Check sheet for the drawn part. Datum: minimum x, y, z corner. Units: mm. A direction names the side the tool comes from. Give positions to 0.01 mm unless a question says otherwise; leave off trailing zeros. Write each loop counter-clockwise with the first axis right and the second up, starting at its lowest first coordinate (ties: lowest second). Pieces come first, ordered by that corner, then holes. Notation, with made-up numbers: (66.5, 31.25) - (117.5, 31.25) arc R30 ccw to (117.5, 61.25) - close; hole circle Ø10 at (-26, 16). An arc over 180 degrees is marked (long way). Use a Markdown table: item, result.
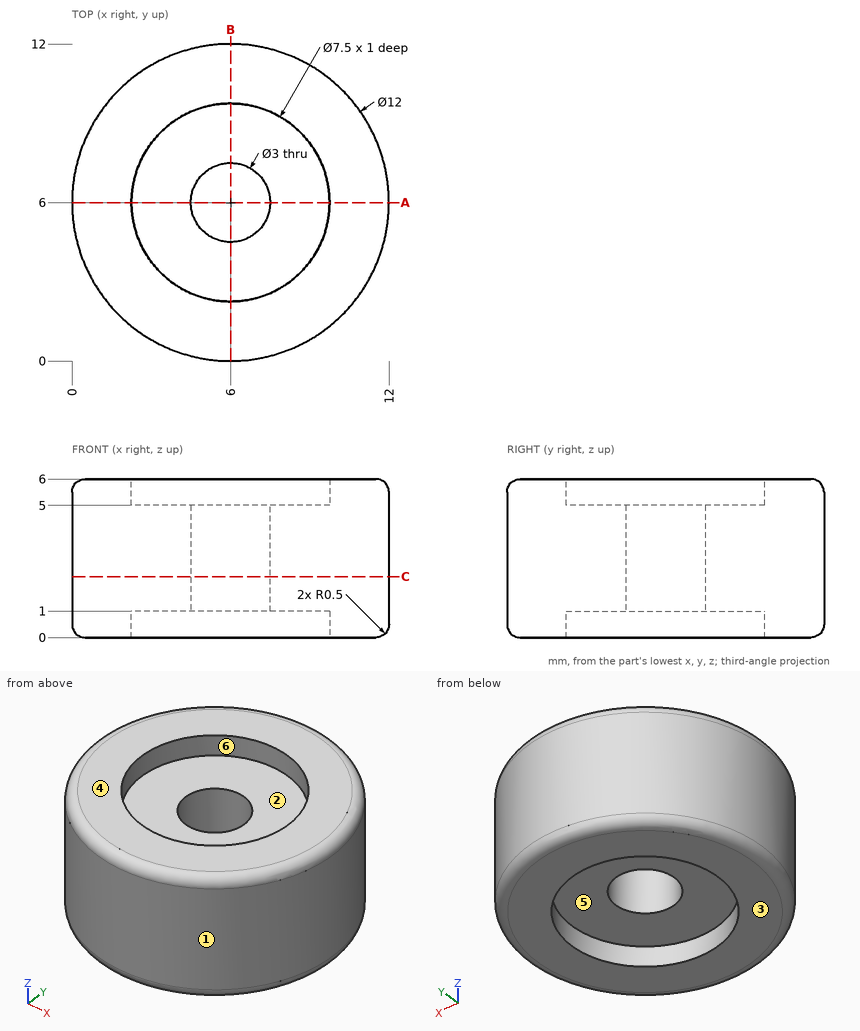
1) Material ranges on L1, parallel to Y at x = 6, z = 0.7; L2, parallel to Y at x = 6, z = 2.5; L3, parallel to Z at x = 9, y = 5.5, recorded low to high. Write a range as from..to.
Working result:
| item | result |
|---|---|
| L1 | y = 0..2.25, 9.75..12 |
| L2 | y = 0..4.5, 7.5..12 |
| L3 | z = 1..5 |
2) Mould release check, pull along X, two halves, no side actions. Record for the marked faces 1, 2 and 3: pulls with the +X half, pulls with the -X half, needs draft (parallel to the pull), parting line crosses it, or undercut.
Working result:
| item | result |
|---|---|
| face 1 | parting line crosses it |
| face 2 | undercut |
| face 3 | needs draft |
3) Section check A-A on y = 6. Record the boundary of the cut face in (x, z).
Working result:
| item | result |
|---|---|
| outline | (0, 0.5) arc R0.5 ccw to (0.5, 0) - (2.25, 0) - (2.25, 1) - (4.5, 1) - (4.5, 5) - (2.25, 5) - (2.25, 6) - (0.5, 6) arc R0.5 ccw to (0, 5.5) - close; (7.5, 1) - (9.75, 1) - (9.75, 0) - (11.5, 0) arc R0.5 ccw to (12, 0.5) - (12, 5.5) arc R0.5 ccw to (11.5, 6) - (9.75, 6) - (9.75, 5) - (7.5, 5) - close |
4) Set-up check for the marked faces 4, 5 and 6: record each of +Z, -Z, +X, -X, +Y, -Y from which the full face is reachable in a straight line by a thin tool's end or side.
Working result:
| item | result |
|---|---|
| face 4 | +Z, +X, -X, +Y, -Y |
| face 5 | -Z |
| face 6 | +Z |
5) Depth check by flat-ended pin: P1, Ø2, axis at x = 2.5, z = 1.5, coming from the -Y side; P2, Ø7, axis at x = 6, y = 6, coming from the -Z side; P3, Ø2.5, axis at x = 6, y = 6, coming from the +Z side. Enter the tip coordinate at first touch or a pass-through.
Working result:
| item | result |
|---|---|
| P1 | stops at y = 0.55 |
| P2 | stops at z = 1 |
| P3 | passes through |
6) Section check C-C on z = 2.3. Record the boundary of the cut face in (x, y).
Working result:
| item | result |
|---|---|
| outline | circle Ø12 at (6, 6); hole circle Ø3 at (6, 6) |
